Can you work these out from the drawing? Everything is in mm from the part's minimum corner. Coordinates: 2 decimals unless noted, no trailing zeros. Write each loop counter-clockwise with the first axis right and the second up, starting at its lowest first coordinate (ties: lowest second). Pieces come first, ordered by that corner, then holes. Notation, with made-up numbers: (0.5, -11) -> (34.5, -11) arc R36 cw to (34.5, 26) -> close; hole circle Ø1 at (26, -11.75). An arc over 180 degrees is marked (long way). Use a Markdown table: item, result. Add a question column.
Item 1: Imagine slicing it at C-C, the plane y = 1.5. Write out the boundary of the cut face in (x, z).
Item 2: Imagine slicing it at B-B, the plane x = 2. Write out the boundary of the cut face in (y, z) (1 decimal).
Item 3: If I drill on line 1 along X through (y, z) = (2, 0.1) (1 decimal); line 2 along X through (y, z) = (4, 0.2); line 3 along Y through (x, z) = (21.5, 0.15) (1 decimal), over which ranges is the centre line in solid material (lowest first)? Write a range as from..to.
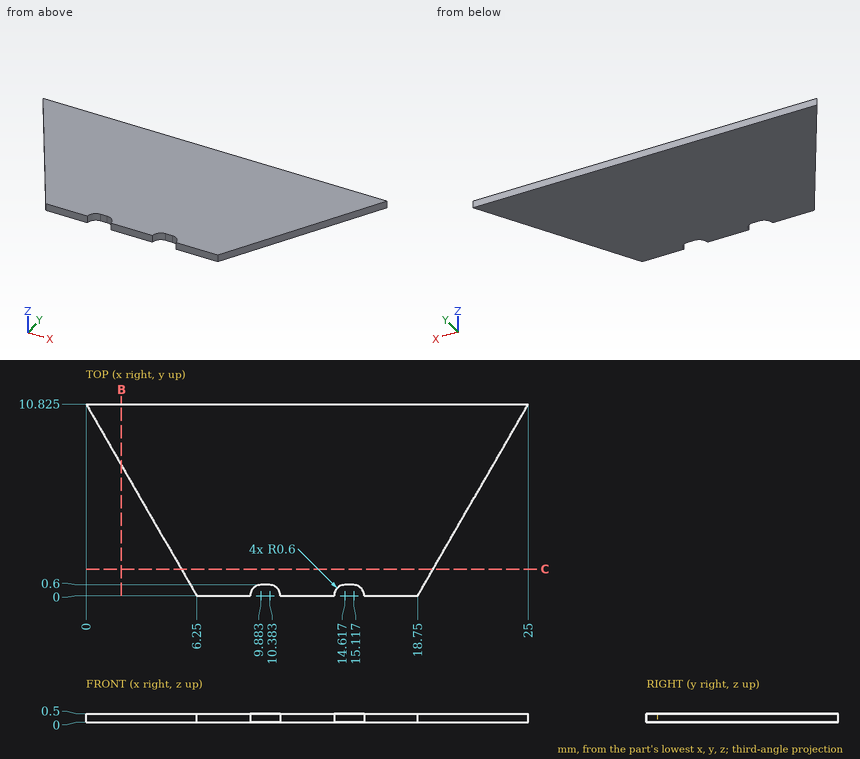
Ans:
| question | item | result |
|---|---|---|
| 1 | outline | (5.38, 0) -> (19.62, 0) -> (19.62, 0.5) -> (5.38, 0.5) -> close |
| 2 | outline | (7.4, 0) -> (10.8, 0) -> (10.8, 0.5) -> (7.4, 0.5) -> close |
| 3 | line 1 | x = 5.1..19.9 |
| 3 | line 2 | x = 3.94..21.06 |
| 3 | line 3 | y = 4.8..10.8 |
